Check sheet for the drawn part. Datum: minimum x, y, z corner. Units: mm. A direction names the side the tool comes from. Give positions to 0.01 mm unless a question says otherwise; leave off trailing zeros. Loops run counter-clockwise (first coordinate to the right, second up) from the corner with the lowest first, then second, coordinate; pieces in that order, holes last.
1. Release check for a two-part mould opening along X. For the marked faces 1, 2, 3 and 4 record: +X half, -X half, draft (parallel to the pull), parting line (faces both ways), or undercut.
2. Cross-section at B-B, the plane z = 12.5. Record the cut outline in (x, y), plus the area to 3 significant figures.
3. Cross-section at A-A, the plane x = 45. Record the cut outline in (y, z) (1 decimal).
4. Material ranges on L1, parallel to Y at x = 97, z = 37.5; L2, parallel to X at y = 40, z = 27; L3, parallel to X at y = 5, z = 24.5 (1 decimal), recorded low to high.
5. Go/stop test with flat-tipped pins: pin 1 Ø1 at (x, y) = (67, 14) entering from +Z; pin 2 Ø5 at (x, z) = (18.5, 17) entering from -Y; pin 3 Ø8 at (x, y) = (27, 18) entering from +Z (1 decimal). Record where each tip stops, or that it passes through.
6. Cross-section at C-C, the plane y = 20. Record the cut outline in (x, z).
7. Tool access check on the marked faces 5 and 6. Record the directions out of +Z, -Z, +X, -X, +Y, -Y that give a thin tool (end or side, any length) a straight path to the whole face; none if there is none.
8. Cross-section at D-D, the plane x = 33.5. Record the cut outline in (y, z) (1 decimal), plus the area to 3 significant figures.
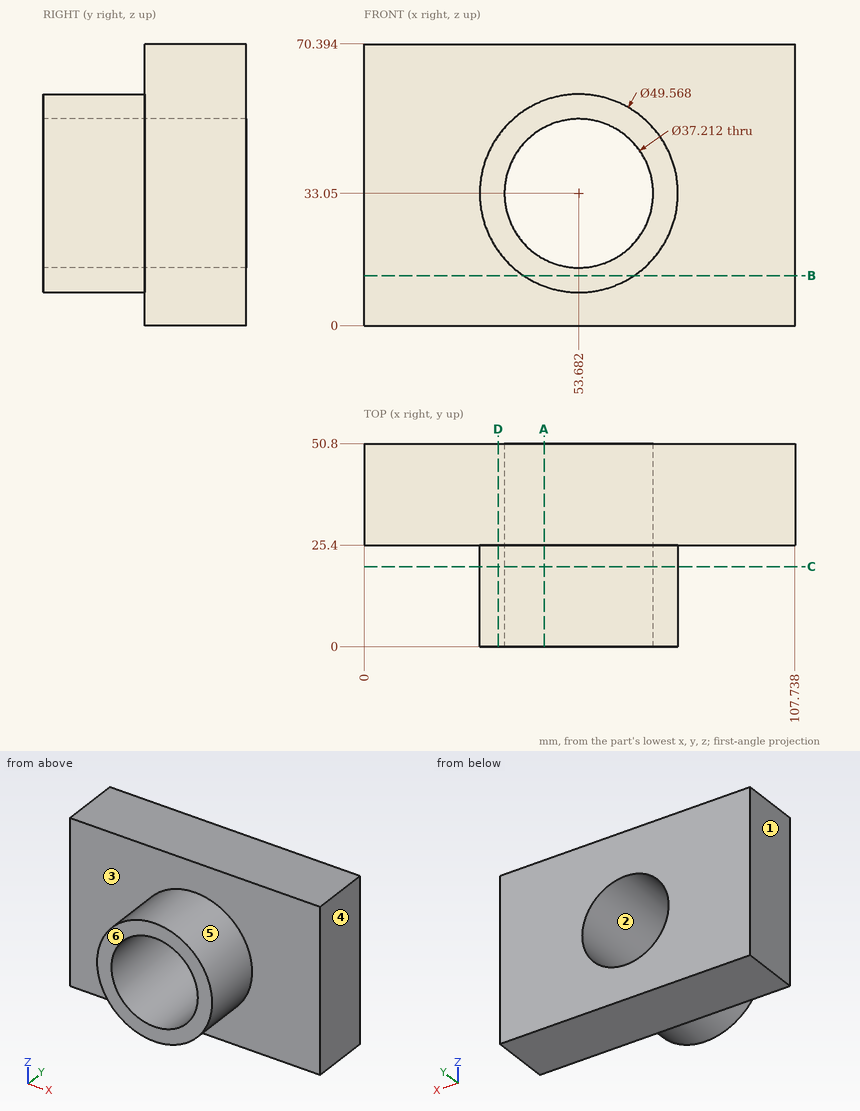
Result:
1. face 1: -X half
1. face 2: undercut
1. face 3: draft
1. face 4: +X half
2. outline: (0, 25.4) - (39.83, 25.4) - (39.83, 0) - (67.54, 0) - (67.54, 25.4) - (107.74, 25.4) - (107.74, 50.8) - (0, 50.8) - close
2. area: 3,440 mm2
3. outline: (0, 9.8) - (25.4, 9.8) - (25.4, 0) - (50.8, 0) - (50.8, 16.6) - (0, 16.6) - close; (0, 49.5) - (50.8, 49.5) - (50.8, 70.4) - (25.4, 70.4) - (25.4, 56.3) - (0, 56.3) - close
4. L1: y = 25.4 to 50.8
4. L2: x = 0 to 36.09, 71.28 to 107.74
4. L3: x = 30.4 to 37.2, 70.2 to 76.9
5. pin 1: stops at z = 54.26
5. pin 2: stops at y = 25.4
5. pin 3: stops at z = 43
6. outline: circle Ø49.57 at (53.68, 33.05); hole circle Ø37.21 at (53.68, 33.05)
7. face 5: -Y
7. face 6: +Z, -Z, +X, -X, -Y
8. outline: (0, 18.7) - (25.4, 18.7) - (25.4, 0) - (50.8, 0) - (50.8, 70.4) - (25.4, 70.4) - (25.4, 47.4) - (0, 47.4) - close
8. area: 2,520 mm2
